from build123d import *
from build123d.topology import SkipClean

# Parameters (mm, degrees)
BOSS_EXTRUDE1_DEPTH = 3
CUT_EXTRUDE1_DEPTH  = 10
CUT_EXTRUDE3_START  = 8
SKETCH8_W           = 6
SKETCH8_H           = 3
CUT_EXTRUDE3_DEPTH  = 6
BOSS_EXTRUDE4_START = 18
BOSS_EXTRUDE4_DEPTH = 28
BOSS_EXTRUDE5_DEPTH = 3
CUT_EXTRUDE4_DEPTH  = 3
CHAMFER1_SIZE       = 15
CHAMFER2_SIZE       = 15
CHAMFER2_SIZE_2     = 10.503113073
CUT_EXTRUDE5_DEPTH  = 10
CUT_EXTRUDE6_DEPTH  = 5
BOSS_EXTRUDE8_DEPTH = 2
CHAMFER3_DEPTH      = 4
CHAMFER3_2_DEPTH    = 3


with BuildPart() as part:
    # Sketch1 → Boss-Extrude1 (new body)
    with BuildSketch(Plane(origin=(0, 0, 0), x_dir=(1, 0, 0), z_dir=(0, 1, 0))):
        with BuildLine():
            ThreePointArc((-49, -6), (-53.242640687, -4.242640687), (-55, 0))
            ThreePointArc((-55, 0), (-51.485281374, -8.485281374), (-43, -12))
            Line((-43, -12), (43, -12))
            ThreePointArc((43, -12), (51.485281374, -8.485281374), (55, 0))
            ThreePointArc((55, 0), (53.242640687, -4.242640687), (49, -6))
            Line((49, -6), (-49, -6))
        make_face()
        with BuildLine():
            Line((-53, 0), (-55, 0))
            ThreePointArc((-55, 0), (-53.242640687, -4.242640687), (-49, -6))
            Line((-49, -6), (49, -6))
            ThreePointArc((49, -6), (53.242640687, -4.242640687), (55, 0))
            Line((55, 0), (53, 0))
            ThreePointArc((53, 0), (51.5, -1.5), (50, 0))
            Line((50, 0), (-50, 0))
            ThreePointArc((-50, 0), (-51.5, -1.5), (-53, 0))
        make_face()
        with BuildLine():
            Line((49, 6), (-49, 6))
            ThreePointArc((-49, 6), (-53.242640687, 4.242640687), (-55, 0))
            Line((-55, 0), (-53, 0))
            ThreePointArc((-53, 0), (-51.5, 1.5), (-50, 0))
            Line((-50, 0), (50, 0))
            ThreePointArc((50, 0), (51.5, 1.5), (53, 0))
            Line((53, 0), (55, 0))
            ThreePointArc((55, 0), (53.242640687, 4.242640687), (49, 6))
        make_face()
    extrude(amount=BOSS_EXTRUDE1_DEPTH)

    # Sketch2 → Cut-Extrude1 (cut)
    with BuildSketch(Plane(origin=(0, 3, 0), x_dir=(1, 0, 0), z_dir=(0, 1, 0))):
        Polygon((22, -8), (36, 6), (-14, 6), (0, -8), align=None)
    extrude(amount=-CUT_EXTRUDE1_DEPTH, mode=Mode.SUBTRACT)

    # Sketch8 → Cut-Extrude3 (cut)
    with BuildSketch(Plane.XY.offset(CUT_EXTRUDE3_START)):
        with Locations((10.960071178, 1.5)):
            Rectangle(SKETCH8_W, SKETCH8_H)
    extrude(amount=CUT_EXTRUDE3_DEPTH, mode=Mode.SUBTRACT)


with BuildPart() as cut_extrude3_piece_1:
    # of the separate pieces the step leaves, piece 1, a body of its own (cut_extrude3_pieces)
    add(part.part.solids().sort_by_distance((-55, 0, 0))[0])

    # Sketch9 → Boss-Extrude4 (add)
    with BuildSketch(Plane(origin=(0, 0, 0), x_dir=(1, 0, 0), z_dir=(0, 1, 0)).offset(BOSS_EXTRUDE4_START)):
        Polygon((13.960071178, -11.2), (13.960071178, -8), (14.760071178, -8), (14.760071178, -12), (7.160071178, -12), (7.160071178, -8), (7.960071178, -8), (7.960071178, -11.2), align=None)
    extrude(amount=-BOSS_EXTRUDE4_DEPTH)


with BuildPart() as cut_extrude3_piece_2:
    # of the separate pieces the step leaves, piece 2, a body of its own (cut_extrude3_pieces)
    add(part.part.solids().sort_by_distance((13.960071178, 0, 12))[0])


with BuildPart() as cut_extrude3_piece_1_1:
    add(cut_extrude3_piece_1.part)

    # Combine1: union Cut-Extrude3 piece 2
    add(cut_extrude3_piece_2.part)

    # Sketch11 → Boss-Extrude5 (add)
    with BuildSketch(Plane(origin=(0, 3, 0), x_dir=(1, 0, 0), z_dir=(0, 1, 0))):
        Polygon((-14, 6), (-12, 6), (2, -8), (0, -8), align=None)
        Polygon((20, -8), (34, 6), (36, 6), (22, -8), align=None)
    extrude(amount=-BOSS_EXTRUDE5_DEPTH)

    # Sketch13 → Cut-Extrude4 (cut)
    with BuildSketch(Plane(origin=(0, 3, 0), x_dir=(1, 0, 0), z_dir=(0, 1, 0))):
        Polygon((2, -8), (-2, -8), (-2, -4), align=None)
        Polygon((24, -4), (24, -8), (20, -8), align=None)
    extrude(amount=-CUT_EXTRUDE4_DEPTH, mode=Mode.SUBTRACT)

    # Chamfer1
    chamfer1_edges = [cut_extrude3_piece_1_1.edges().sort_by_distance(p)[0] for p in [
        (14.760071178, 3, 10),
        (7.160071178, 3, 10),
    ]]
    chamfer(chamfer1_edges, length=CHAMFER1_SIZE - 0.0001)  # a hair under: the kernel refuses the full size

    # Chamfer2
    # the kernel refuses this chamfer: 15, 10.503113073 mm, written as the material it adds along each edge
    with BuildSketch(Plane(origin=(7.160071178, 0, 12), x_dir=(-1, 0, 0), z_dir=(0, 0, -1))) as chamfer2_piece_1_section:
        Polygon((CHAMFER2_SIZE, 0), (0, -CHAMFER2_SIZE_2), (0, 0), align=None)
    chamfer2_piece_1 = extrude(amount=4, mode=Mode.PRIVATE)
    chamfer2_piece_1 = split(chamfer2_piece_1, bisect_by=Plane(origin=(-2, 0, 12), z_dir=(-1, 0, 0)), keep=Keep.TOP, mode=Mode.PRIVATE)
    add(chamfer2_piece_1)
    with BuildSketch(Plane(origin=(7.160071178, 0, 12), x_dir=(-1, 0, 0), z_dir=(0, 0, -1))) as chamfer2_piece_2_section:
        Polygon((CHAMFER2_SIZE, 0), (0, -CHAMFER2_SIZE_2), (0, 0), align=None)
    chamfer2_piece_2 = extrude(amount=4, mode=Mode.PRIVATE)
    chamfer2_piece_2 = split(chamfer2_piece_2, bisect_by=Plane(origin=(6.580035589, 0, 12.580035589), z_dir=(-0.7071067811865489, 0, 0.7071067811865461)), keep=Keep.TOP, mode=Mode.PRIVATE)
    chamfer2_piece_2 = split(chamfer2_piece_2, bisect_by=Plane(origin=(-2, 0, 12), z_dir=(1, 0, 0)), keep=Keep.TOP, mode=Mode.PRIVATE)
    add(chamfer2_piece_2)
    with BuildSketch(Plane(origin=(7.160071178, 0, 12), x_dir=(-1, 0, 0), z_dir=(0, 0, -1))) as chamfer2_piece_3_section:
        Polygon((CHAMFER2_SIZE, 0), (0, -CHAMFER2_SIZE_2), (0, 0), align=None)
    chamfer2_piece_3 = extrude(amount=42.738283454, mode=Mode.PRIVATE)
    chamfer2_piece_3 = split(chamfer2_piece_3, bisect_by=Plane(origin=(6.580035589, 0, 12.580035589), z_dir=(-0.7071067811865489, 0, 0.7071067811865461)), keep=Keep.TOP, mode=Mode.PRIVATE)
    chamfer2_piece_3 = split(chamfer2_piece_3, bisect_by=Plane(origin=(-2, 0, 12), z_dir=(-1, 0, 0)), keep=Keep.TOP, mode=Mode.PRIVATE)
    chamfer2_piece_3 = split(chamfer2_piece_3, bisect_by=Plane(origin=(7.160071178, 0, 8), z_dir=(0, 0, -1)), keep=Keep.TOP, mode=Mode.PRIVATE)
    add(chamfer2_piece_3)
    with BuildSketch(Plane(origin=(7.160071178, 0, 12), x_dir=(-1, 0, 0), z_dir=(0, 0, -1))) as chamfer2_piece_4_section:
        Polygon((CHAMFER2_SIZE, 0), (0, -CHAMFER2_SIZE_2), (0, 0), align=None)
    chamfer2_piece_4 = extrude(amount=4, mode=Mode.PRIVATE)
    chamfer2_piece_4 = split(chamfer2_piece_4, bisect_by=Plane(origin=(6.580035589, 0, 12.580035589), z_dir=(0.7071067811865489, 0, -0.7071067811865461)), keep=Keep.TOP, mode=Mode.PRIVATE)
    chamfer2_piece_4 = split(chamfer2_piece_4, bisect_by=Plane(origin=(7.160071178, -10, 12), z_dir=(0, 1, 0)), keep=Keep.TOP, mode=Mode.PRIVATE)
    add(chamfer2_piece_4)
    with BuildSketch(Plane(origin=(14.760071178, 0, 12), x_dir=(0, -1, 0), z_dir=(0, 0, -1))) as chamfer2_piece_5_section:
        Polygon((CHAMFER2_SIZE_2, 0), (0, -CHAMFER2_SIZE), (0, 0), align=None)
    chamfer2_piece_5 = extrude(amount=4, mode=Mode.PRIVATE)
    chamfer2_piece_5 = split(chamfer2_piece_5, bisect_by=Plane(origin=(15.380035589, 0, 12.619964411), z_dir=(0.7071067811865462, 0, 0.7071067811865489)), keep=Keep.TOP, mode=Mode.PRIVATE)
    chamfer2_piece_5 = split(chamfer2_piece_5, bisect_by=Plane(origin=(24, 0, 12), z_dir=(-1, 0, 0)), keep=Keep.TOP, mode=Mode.PRIVATE)
    add(chamfer2_piece_5)
    with BuildSketch(Plane(origin=(14.760071178, 0, 12), x_dir=(0, -1, 0), z_dir=(0, 0, -1))) as chamfer2_piece_6_section:
        Polygon((CHAMFER2_SIZE_2, 0), (0, -CHAMFER2_SIZE), (0, 0), align=None)
    chamfer2_piece_6 = extrude(amount=4, mode=Mode.PRIVATE)
    chamfer2_piece_6 = split(chamfer2_piece_6, bisect_by=Plane(origin=(24, 0, 12), z_dir=(1, 0, 0)), keep=Keep.TOP, mode=Mode.PRIVATE)
    add(chamfer2_piece_6)
    with BuildSketch(Plane(origin=(14.760071178, 0, 12), x_dir=(0, -1, 0), z_dir=(0, 0, -1))) as chamfer2_piece_7_section:
        Polygon((CHAMFER2_SIZE_2, 0), (0, -CHAMFER2_SIZE), (0, 0), align=None)
    chamfer2_piece_7 = extrude(amount=4, mode=Mode.PRIVATE)
    chamfer2_piece_7 = split(chamfer2_piece_7, bisect_by=Plane(origin=(14.760071178, -10, 12), z_dir=(0, 1, 0)), keep=Keep.TOP, mode=Mode.PRIVATE)
    chamfer2_piece_7 = split(chamfer2_piece_7, bisect_by=Plane(origin=(15.380035589, 0, 12.619964411), z_dir=(-0.7071067811865462, 0, -0.7071067811865489)), keep=Keep.TOP, mode=Mode.PRIVATE)
    add(chamfer2_piece_7)
    with BuildSketch(Plane(origin=(14.760071178, 0, 12), x_dir=(0, -1, 0), z_dir=(0, 0, -1))) as chamfer2_piece_8_section:
        Polygon((CHAMFER2_SIZE_2, 0), (0, -CHAMFER2_SIZE), (0, 0), align=None)
    chamfer2_piece_8 = extrude(amount=42.738283454, mode=Mode.PRIVATE)
    chamfer2_piece_8 = split(chamfer2_piece_8, bisect_by=Plane(origin=(14.760071178, 0, 8), z_dir=(0, 0, -1)), keep=Keep.TOP, mode=Mode.PRIVATE)
    chamfer2_piece_8 = split(chamfer2_piece_8, bisect_by=Plane(origin=(15.380035589, 0, 12.619964411), z_dir=(0.7071067811865462, 0, 0.7071067811865489)), keep=Keep.TOP, mode=Mode.PRIVATE)
    chamfer2_piece_8 = split(chamfer2_piece_8, bisect_by=Plane(origin=(24, 0, 12), z_dir=(1, 0, 0)), keep=Keep.TOP, mode=Mode.PRIVATE)
    add(chamfer2_piece_8)

    # Sketch15 → Cut-Extrude5 (cut)
    with BuildSketch(Plane.XY.offset(12)):
        with BuildLine():
            Line((14.160071178, 12.5), (14.160071178, -4.5))
            ThreePointArc((14.160071178, -4.5), (10.960071178, -7.7), (7.760071178, -4.5))
            Line((7.760071178, -4.5), (7.760071178, 12.5))
            ThreePointArc((7.760071178, 12.5), (10.960071178, 15.7), (14.160071178, 12.5))
        make_face()
    extrude(amount=-CUT_EXTRUDE5_DEPTH, mode=Mode.SUBTRACT)

    # Sketch16 → Cut-Extrude6 (cut)
    with BuildSketch(Plane(origin=(0, 0, 0), x_dir=(1, 0, 0), z_dir=(0, 1, 0))):
        Polygon((-7.839928822, 1.839928822), (-2, -4), (-2, -7.160071178), (-7.839928822, -7.160071178), align=None)
        Polygon((24, -7.160071178), (24, -4), (29.760071178, 1.760071178), (29.760071178, -7.160071178), align=None)
    extrude(amount=-CUT_EXTRUDE6_DEPTH, mode=Mode.SUBTRACT)

    # Sketch17 → Boss-Extrude8 (add)
    with SkipClean():  # the faces are left unmerged after this step: merging them gives an invalid solid
        with BuildSketch(Plane.XY.offset(12)):
            Polygon((-7.839928822, 0), (6.441551245, -10), (15.47859111, -10), (29.760071178, 0), (43, 0), (43, 3), (29.760071178, 3), (14.760071178, 18), (7.160071178, 18), (-7.839928822, 3), (-43, 3), (-43, 0), align=None)
            with BuildLine():
                Line((7.760071178, -4.5), (7.760071178, 12.5))
                ThreePointArc((7.760071178, 12.5), (10.960071178, 15.7), (14.160071178, 12.5))
                Line((14.160071178, 12.5), (14.160071178, -4.5))
                ThreePointArc((14.160071178, -4.5), (10.960071178, -7.7), (7.760071178, -4.5))
            make_face(mode=Mode.SUBTRACT)
        extrude(amount=BOSS_EXTRUDE8_DEPTH)

    # Chamfer3: read off the stored shape, not the designer's step
    # Chamfer3 outline → Chamfer3 (cut)
    with SkipClean():  # the faces are left unmerged after this step: merging them gives an invalid solid
        with BuildSketch(Plane(origin=(0, 0, 0), x_dir=(1, 0, 0), z_dir=(0, 1, 0))):
            with BuildLine():
                ThreePointArc((47.608318931, -11.079864468), (49.300429772, -10.212961602), (50.834384089, -9.08968789))
                Line((50.834384089, -9.08968789), (47.608318931, -11.079864468))
            make_face()
            with BuildLine():
                ThreePointArc((-50.834384089, -9.08968789), (-49.300429772, -10.212961602), (-47.608318931, -11.079864468))
                Line((-47.608318931, -11.079864468), (-50.834384089, -9.08968789))
            make_face()
        extrude(amount=CHAMFER3_DEPTH, mode=Mode.SUBTRACT)

    # Chamfer3 2 outline → Chamfer3 2 (add)
    with SkipClean():  # the faces are left unmerged after this step: merging them gives an invalid solid
        with BuildSketch(Plane(origin=(0, 0, 0), x_dir=(1, 0, 0), z_dir=(0, 1, 0))):
            with BuildLine():
                Line((43, -13.922760673), (47.608318931, -11.079864468))
                ThreePointArc((47.608318931, -11.079864468), (45.349641077, -11.767717995), (43, -12))
                Line((43, -12), (43, -13.922760673))
            make_face()
            with BuildLine():
                Line((-47.608318931, -11.079864468), (-43, -13.922760673))
                Line((-43, -13.922760673), (-43, -12))
                ThreePointArc((-43, -12), (-45.349641077, -11.767717995), (-47.608318931, -11.079864468))
            make_face()
        extrude(amount=CHAMFER3_2_DEPTH)


solid = cut_extrude3_piece_1_1.part
For this review, take the finished solid that the model builds, in its own axes (mm). A direction names the side the tool comes from. Round coordinates to 2 decimals unless told otherwise and drop trailing zeros. Order: outer loops, then holes, each group sorted by start corner. A loop starts at its lowest first (then second) coordinate and runs counter-clockwise, first axis right, second up. Notation, with made-up numbers: M 58.5,54.5 L 62.5,54.5 A12 cw 62.5,74.5 Z; hole C 72,-18 d1. An arc over 180 degrees is marked long. Use a Markdown table: item, result. Add a question column.
Item 1: Mouldability with a two-part tool opening along X and no side actions: class faces 1 (the flat face through (11, 18, 12)), 2 (the cylindrical face through (-50.3, 1.5, 0.9)), 3 (the cylindrical face through (-53.196, 1.479, -4.289)) as released by +X, released by -X, zero draft, split by the parting line, or undercut.
Item 2: Tool access review of faces 4 (the cylindrical face through (11, -7.7, 12.3)), 5 (the flat face through (11, -9, 11.2)), 6 (the flat face through (-4, -2, 7.16)), 7 (the flat face through (-31, 3, 4)): name each direction out of +Z, -Z, +X, -X, +Y, -Y from which nothing blocks a thin tool from reaching the whole face with its end or side.
Item 3: Insertion check: pin 1 (1.8 mm diameter, centred on y = 1.5, z = 11.5, fed in from -X); pin 2 (3 mm diameter, centred on x = 1.5, y = 4.5, fed in from -Z); pin 3 (11 mm diameter, centred on x = 20, y = 1.5, fed in from -Z). Each pin has a flat end and moves straight along its axis. Give the tip position at first contact, or say it passes through.
Item 4: Add section C-C, the plane x = -39. Give the boundary of the cut face in (y, z).
Item 5: Add section B-B, the plane z = -4. Give the boundary of the cut face in (x, y), then the cut area to 3 significant figures.
Item 6: Add section D-D, the plane x = 26.5. Give the boundary of the cut face in (y, z), then the cut area to 3 significant figures.
Item 7: Add section A-A, the plane y = 2. Give the boundary of the cut face in (x, z), then the cut area to 3 significant figures.
Item 8: To check wall thickness, follow line 1 along X through (y, z) = (1.2, 0); line 2 along Y through (x, z) = (-14.5, 3.25); line 3 along X through (y, z) = (14, 9). State the ranges of each line that lie inside material, in increasing order.
Geometry results:
| question | item | result |
|---|---|---|
| 1 | face 1 | zero draft |
| 1 | face 2 | undercut |
| 1 | face 3 | released by -X |
| 2 | face 4 | +Z, -Z |
| 2 | face 5 | -Z, +Y, -Y |
| 2 | face 6 | -Z, +X, -X, -Y |
| 2 | face 7 | +Z, -Z, -X, +Y |
| 3 | pin 1 | stops at x = -48.39 |
| 3 | pin 2 | stops at z = 8 |
| 3 | pin 3 | stops at z = 2.5 |
| 4 | outline | M 0,-6 L 3,-6 L 3,14 L 0,14 Z |
| 5 | outline | M -53.47,0 L -10,0 L -10,3 L -53.47,3 Z; M 32,0 L 53.47,0 L 53.47,3 L 32,3 Z |
| 5 | area | 195 mm² |
| 6 | outline | M -2.28,7.16 L 0,7.16 L 0,1.5 L 6.26,1.5 L 6.26,14 L -2.28,14 Z |
| 6 | area | 93.9 mm² |
| 7 | outline | M -55,0 A6 ccw -49,-6 L -12,-6 L -2,4 L -2,8 L 7.76,8 L 7.76,14 L -43,14 L -43,13.92 L -50.83,9.09 A12 ccw Z; M 14.16,8 L 24,8 L 24,4 L 34,-6 L 49,-6 A6 ccw 55,0 A12 ccw 50.83,9.09 L 43,13.92 L 43,14 L 14.16,14 Z; hole C -51.5,0 d3; hole C 51.5,0 d3 |
| 7 | area | 1,560 mm² |
| 8 | line 1 | x = -55 to -53, -50 to -6, 28 to 50, 53 to 55 |
| 8 | line 2 | y = 0 to 3 |
| 8 | line 3 | x = 3.16 to 7.96, 13.96 to 18.76 |
